from build123d import *

# Parameters (mm, degrees)
SKETCH1_R                    = 25
BOSS_EXTRUDE1_DEPTH          = 2
SKETCH2_W                    = 20
SKETCH2_H                    = 2
CUT_EXTRUDE_THIN1_DEPTH      = 1
CUT_EXTRUDE_THIN1_DEPTH_BACK = 1


with BuildPart() as part:
    # Sketch1 → Boss-Extrude1 (new body)
    with BuildSketch(Plane(origin=(0, 0, 0), x_dir=(1, 0, 0), z_dir=(0, 1, 0))):
        Circle(SKETCH1_R)
    extrude(amount=BOSS_EXTRUDE1_DEPTH)

    # Sketch2 → Cut-Extrude-Thin1 (cut, two sides)
    with BuildSketch(Plane(origin=(0, 2, 0), x_dir=(1, 0, 0), z_dir=(0, 1, 0))) as cut_extrude_thin1_sk:
        with Locations((10, 0)):
            Rectangle(SKETCH2_W, SKETCH2_H)
    extrude(amount=CUT_EXTRUDE_THIN1_DEPTH, mode=Mode.SUBTRACT)
    extrude(cut_extrude_thin1_sk.sketch, amount=-CUT_EXTRUDE_THIN1_DEPTH_BACK, mode=Mode.SUBTRACT)


solid = part.part
Can you work these out from the model? Positions are in its coordinate system, mm. Give positions to 0.01 mm unless a question says otherwise; leave off trailing zeros. Loops run counter-clockwise (first coordinate to the right, second up) from the corner with the lowest first, then second, coordinate; pieces in that order, holes last. Notation, with made-up numbers: (76.25, 10.25) - (127.25, 10.25) arc R6 cw to (127.25, 20.25) - close; hole circle Ø4 at (66, 51.5). An arc over 180 degrees is marked (long way). Return JSON: item names as keys, results as strings.
1. I want a section at C-C on x = 3. Please give me the cut outline in (y, z), and give its area (3 significant figures).
Output values:
{"outline": "(0, -24.82) - (2, -24.82) - (2, -1) - (1, -1) - (1, 1) - (2, 1) - (2, 24.82) - (0, 24.82) - close", "area": "97.3 mm²"}
2. I want a section at D-D on z = 6. Please give me the cut outline in (x, y), and give its area (3 significant figures).
Output values:
{"outline": "(-24.27, 0) - (24.27, 0) - (24.27, 2) - (-24.27, 2) - close", "area": "97.1 mm²"}
3. I want a section at A-A on z = 0. Please give me the cut outline in (x, y), and give its area (3 significant figures).
Output values:
{"outline": "(-25, 0) - (25, 0) - (25, 2) - (20, 2) - (20, 1) - (0, 1) - (0, 2) - (-25, 2) - close", "area": "80.0 mm²"}
4. I'm going to push flat-ended pins straight in: pin 1 Ø0.5 at (x, y) = (10.5, 1.5) entering from -Z; pin 2 Ø0.8 at (x, y) = (8, 1.5) entering from +Z. Where does each tip first touch, or does it pass through?
Output values:
{"pin 1": "stops at z = -22.8", "pin 2": "stops at z = 23.82"}
5. If I drill on line 1 (Z direction, x = 3.5, y = 1.9); line 2 (Z direction, x = 8, y = 1.85); line 3 (Z direction, x = 9, y = 0.7), over which ranges is the centre line in solid material (lowest first)?
Output values:
{"line 1": "z = -24.75 to -1, 1 to 24.75", "line 2": "z = -23.69 to -1, 1 to 23.69", "line 3": "z = -23.32 to 23.32"}
6. I want a section at B-B on y = 1.55. Please give me the cut outline in (x, z), and give its area (3 significant figures).
Output values:
{"outline": "circle Ø50 at (0, 0); hole (0, -1) - (20, -1) - (20, 1) - (0, 1) - close", "area": "1,920 mm²"}
7. We'd pull the mould along X, two halves only. Please class faces 1 (the face through (23.846, 0.986, -7.509)), 2 (the face through (10, 1, 0)), 3 (the face through (0, 0, 0)): +X half, -X half, draft (parallel to the pull), parting line (faces both ways), or undercut.
Output values:
{"face 1": "parting line", "face 2": "undercut", "face 3": "draft"}
